from build123d import *

# Parameters (mm, degrees)
F2_R     = 6.35
F4_DEPTH = 127


with BuildPart() as f1:
    # F0 (on Front) → F1 (revolve)
    with BuildSketch(Plane.XZ):
        with BuildLine():
            ThreePointArc((-21.799631, 61.9125), (-19.87175, 57.258186), (-15.875, 60.325))
            ThreePointArc((-15.875, 60.325), (-16.804936, 62.570064), (-19.05, 63.5))
            ThreePointArc((-19.05, 63.5), (-20.6375, 63.074631), (-21.799631, 61.9125))
        make_face()
        with BuildLine():
            Line((-36.5125, 0), (-15.875, 0))
            Line((-15.875, 0), (-15.875, 60.325))
            ThreePointArc((-15.875, 60.325), (-19.87175, 57.258186), (-21.799631, 61.9125))
            Line((-21.799631, 61.9125), (-36.5125, 36.429063))
            Line((-36.5125, 36.429063), (-36.5125, 0))
        make_face()
    revolve(axis=Axis((0, 0, 26.929792), (0, 0, 1)))

    # F2
    f2_edges = [f1.edges().sort_by_distance(p)[0] for p in [
        (36.5125, 0, 36.429063),
    ]]
    fillet(f2_edges, radius=F2_R)

    # F3 (on Front) → F4 (cut, symmetric)
    with BuildSketch(Plane.XZ):
        Polygon((0, 88.9), (0, 63.5), (50.8, 12.7), (50.8, 88.9), align=None)
    extrude(amount=F4_DEPTH, both=True, mode=Mode.SUBTRACT)


solid = f1.part
Source: CAD feature listing. Evaluate the final solid. Frame: model axes, mm. Round coordinates to 2 decimals unless told otherwise and drop trailing zeros. Order: outer loops, then holes, each group sorted by start corner. A loop starts at its lowest first (then second) coordinate and runs counter-clockwise, first axis right, second up. Notation, with made-up numbers: (-19, 11.5) -> (-9, 11.5) arc R12 cw to (-9, 26.5) -> close; hole circle Ø6 at (-0.75, -2.5). An arc over 180 degrees is marked (long way). Answer as CSV lines item,"result".
Item 1: Section C-C, the plane z = 56.5. Return loops of the section in (x, y) (3 decimals), plus the area to 3 significant figures.
A:
outline,"(7, -23.921) -> (7, -14.248) arc R15.875 cw (long way) to (7, 14.248) -> (7, 23.921) arc R24.925 ccw (long way) to start"
area,"709 mm²"
Item 2: Pull-direction query (X, two-part tool) for faces 1 (the face through (-14.664, 6.08, 30.585)), 2 (the face through (-34.826, -10.967, 17.121)), 3 (the face through (-16, 8, 0)), 4 (the face through (22.1, -0.4, 41.4)); classes: pulls with the +X half, pulls with the -X half, needs draft (parallel to the pull), parting line crosses it, or undercut.
A:
face 1,"undercut"
face 2,"parting line crosses it"
face 3,"needs draft"
face 4,"pulls with the +X half"
Item 3: Pin query (flat end, axial travel): pin 1 Ø8 at (x, z) = (28.5, 37.5) entering from +Y; pin 2 Ø1.5 at (y, z) = (24, 16) entering from -X; pin 3 Ø8 at (y, z) = (27.5, 27) entering from -X. Return the tip coordinate at first contact, or that it passes through.
A:
pin 1,"y = 26.64"
pin 2,"x = -28.15"
pin 3,"x = -27.94"
Item 4: Section B-B, the plane x = 32.5. Return loops of the section in (y, z), plus the area to 3 significant figures.
A:
outline,"(-16.64, 0) -> (16.64, 0) -> (16.64, 31) -> (-16.64, 31) -> close"
area,"1,030 mm²"
Item 5: Line query: L1, parallel to Y at x = 0, z = 23 (1 decimal); L2, parallel to Y at x = -16.5, z = 60. Output: solid intervals per line, ascending.
A:
L1,"-36.5 to -15.9, 15.9 to 36.5"
L2,"-15.89 to 15.89"
